Study the drawing (mm; zero at the part's minimum x, y, z) and answer. A direction names the side the tool comes from. Coordinates: 2 decimals unless noted, no trailing zeros. Order: outer loops, then holes, each group sorted by start corner. A loop starts at its lowest first (then second) coordinate and runs counter-clockwise, first axis right, second up. Notation, with made-up numbers: (38.5, -10.5) -> (79.5, -10.5) arc R31 cw to (79.5, 23.5) -> close; hole circle Ø7 at (3, 8.25). An arc over 180 degrees is marked (long way). Write each question's results on one line, items separated by ' | '. Start each with the question number.
(1) Determine the mould class of the marked faces 3, 4 and 5 for opening direction Y: +Y half, -Y half, draft (parallel to the pull), parting line (faces both ways), or undercut.
(2) The part is cut by section D-D, the plane y = 11.5. Give the vertices of the cut face in (x, z).
(3) Straight lines are drawn through the part: L1, parallel to Y at x = 26.5, z = 6.5; L2, parallel to X at y = 4, z = 7.75; L3, parallel to X at y = 10, z = 2.25. For each, find the intervals that lie inside material, in ascending order.
(4) The part is cut by section A-A, the plane x = 26.5. Give the vertices of the cut face in (y, z), then the cut area to 3 significant figures.
(5) Given pin 1 (8 mm diameter, centred on y = 3, z = 6.5, fed in from +X); pin 2 (1.5 mm diameter, centred on x = 3.5, z = 11.5, fed in from +Y); pin 3 (10 mm diameter, centred on y = 11.5, z = 5.5, fed in from +X); pin 4 (6 mm diameter, centred on y = 2.5, z = 8, fed in from -X), each flat-ended and moving along its own axis, determine where each tip first touches the part or whether it passes through.
(6) A tool of negligible diameter and unlimited length cuts with its end or side. For the marked faces 1 and 2, from which of +Z, -Z, +X, -X, +Y, -Y can it reach the whole face along a straight path? Write none if from no direction.
(7) The part is cut by section C-C, the plane y = 9.25. Give the vertices of the cut face in (x, z), then the cut area to 3 significant figures.
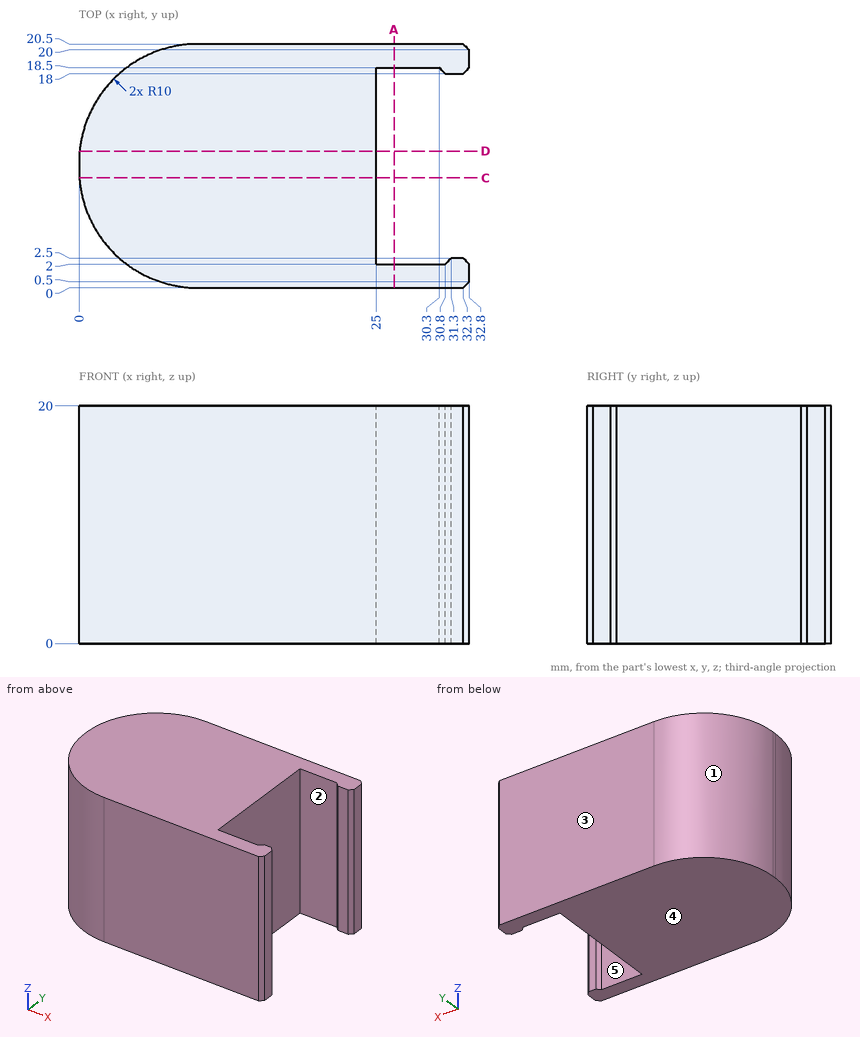
Established:
1) face 3: +Y half | face 4: draft | face 5: undercut
2) outline: (0.05, 0) -> (25, 0) -> (25, 20) -> (0.05, 20) -> close
3) L1: y = 0 to 2, 18.5 to 20.5 | L2: x = 2 to 25 | L3: x = 0 to 25
4) outline: (0, 0) -> (2, 0) -> (2, 20) -> (0, 20) -> close; (18.5, 0) -> (20.5, 0) -> (20.5, 20) -> (18.5, 20) -> close | area: 80.0 mm^2
5) pin 1: stops at x = 32.8 | pin 2: stops at y = 18.68 | pin 3: stops at x = 25 | pin 4: stops at x = 1.07
6) face 1: +Z, -Z, -X, +Y | face 2: +Z, -Z
7) outline: (0.03, 0) -> (25, 0) -> (25, 20) -> (0.03, 20) -> close | area: 499 mm^2
